Source: three-view drawing plus pictorial views. Frame: mm from the lowest corner of the part. Give positions to 0.01 mm unless a question says otherwise; leave off trailing zeros. Order: outer loops, then holes, each group sorted by start corner. A loop starts at its lowest first (then second) coordinate and runs counter-clockwise, first axis right, second up.
1) Section B-B, the plane x = 30.5. Return loops of the section in (y, z).
2) Section A-A, the plane z = 20.75. Return loops of the section in (x, y).
3) First-contact query: P1, Ø2, axis at x = 34, z = 19.5, coming from the +Y side; P2, Ø3, axis at x = 39, z = 4, coming from the -Y side. Flat tips, straight axial feed; report the tip coordinate or a pass-through.
4) Material intervals for line 1 (Y direction, x = 27.5, z = 8.25); line 2 (Y direction, x = 15, z = 4); line 3 (X direction, y = 647.5, z = 23.5), sorted ascending.
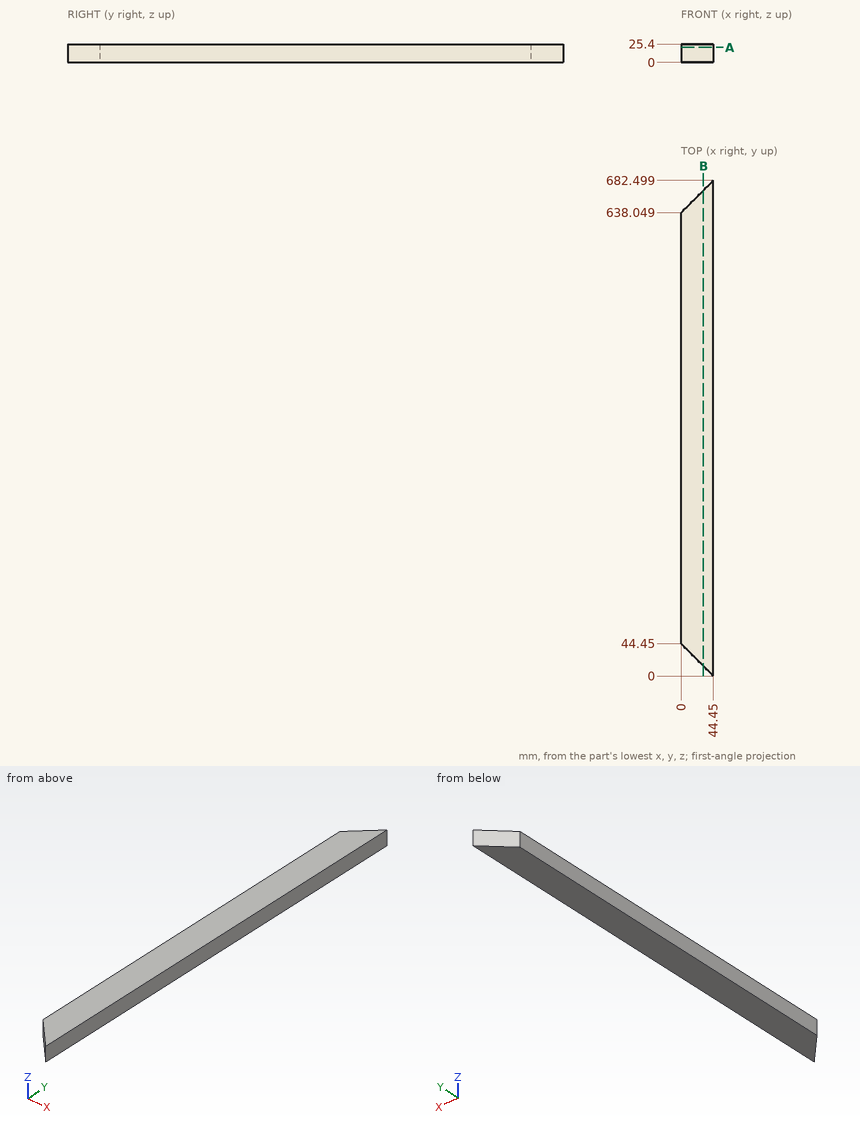
From the geometry:
1. outline: (13.95, 0) - (668.55, 0) - (668.55, 25.4) - (13.95, 25.4) - close
2. outline: (0, 44.45) - (44.45, 0) - (44.45, 682.5) - (0, 638.05) - close
3. P1: stops at y = 673.05
3. P2: stops at y = 3.95
4. line 1: y = 16.95 to 665.55
4. line 2: y = 29.45 to 653.05
4. line 3: x = 9.45 to 44.45
